from build123d import *

# Parameters (mm, degrees)
BOSS_EXTRUDE1_DEPTH = 1.5875
SKETCH2_R           = 13.081
CUT_EXTRUDE1_DEPTH  = 282.7782
CUT_EXTRUDE2_REACH  = 907.396
SKETCH3_R           = 13.081
SKETCH5_RX          = 13.458967046
SKETCH5_RY          = 13.27706685
CUT_EXTRUDE3_DEPTH  = 850.411898389
SKETCH7_RX          = 13.827169688
SKETCH7_RY          = 13.509347203
CUT_EXTRUDE4_DEPTH  = 850.411898525
SURFACECUT1_ANGLE   = 12.730551
CUT_EXTRUDE13_DEPTH = 850.411898527
CUT_EXTRUDE14_START = -3.175
CUT_EXTRUDE14_DEPTH = 3.175
CUT_EXTRUDE15_DEPTH = 850.411898527
CUT_EXTRUDE16_DEPTH = 850.411898527
FILLET1_R           = 25.4
SKETCH28_W          = 101.6
SKETCH28_H          = 1.7907
CUT_EXTRUDE17_DEPTH = 850.411898527
CUT_EXTRUDE18_DEPTH = 850.411898527
CUT_EXTRUDE19_DEPTH = 850.411898527


# Read off the part's stored shape, not the designer's step: SurfaceCut1, Cut-Extrude14
with BuildPart() as part:
    # Sketch1 → Boss-Extrude1 (new, symmetric)
    with BuildSketch(Plane(origin=(-71.4375, 0, 0), x_dir=(0, 0, -1), z_dir=(1, 0, 0))):
        Polygon((139.7, -400.05), (29.21, -400.05), (29.21, -76.2), (-154.94, -76.2), (-154.94, -389.89), (-262.89, -389.89), (-262.89, -76.2), (-384.81, -76.2), (-384.81, -342.9), (-454.66, -342.9), (-454.66, -76.2), (-749.3, -76.2), (-749.3, 76.2), (-454.66, 76.2), (-454.66, 342.9), (-384.81, 342.9), (-384.81, 76.2), (-262.89, 76.2), (-262.89, 389.89), (-154.94, 389.89), (-154.94, 76.2), (29.21, 76.2), (29.21, 400.05), (139.7, 400.05), (139.7, 92.075), (107.95, 92.075), (107.95, 88.9), (139.7, 88.9), (139.7, -88.9), (107.95, -88.9), (107.95, -92.075), (139.7, -92.075), align=None)
    extrude(amount=BOSS_EXTRUDE1_DEPTH, both=True)

    # Sketch2 → Cut-Extrude1 (cut)
    with BuildSketch(Plane(origin=(209.7532, 370.332, -29.3624), x_dir=(0, 0, -1), z_dir=(1, 0, 0))):
        Circle(SKETCH2_R)
    cut_extrude1 = extrude(amount=-CUT_EXTRUDE1_DEPTH, mode=Mode.SUBTRACT)

    # Cut-Extrude2: up to this plane
    cut_extrude2_end = Plane(origin=(-73.025, 0, 0), z_dir=(-1, 0, 0))
    # Sketch3 → Cut-Extrude2 (cut, up to the surface)
    with BuildSketch(Plane(origin=(4.654591859, 367.519252147, 275.4376), x_dir=(0.13291538281760473, 0.03562595760229639, -0.9904868965086662), z_dir=(0.9567163781525703, 0.25643335182849597, 0.13760707774177544)), mode=Mode.PRIVATE) as cut_extrude2_sk1:
        Circle(SKETCH3_R)
    cut_extrude2_tool1 = split(extrude(cut_extrude2_sk1.sketch, amount=-CUT_EXTRUDE2_REACH, mode=Mode.PRIVATE), bisect_by=cut_extrude2_end, keep=Keep.BOTH, mode=Mode.PRIVATE)
    cut_extrude2 = cut_extrude2_tool1.solids().sort_by_distance((4.654592, 367.519252, 275.4376))[0]
    add(cut_extrude2, mode=Mode.SUBTRACT)

    # Sketch5 → Cut-Extrude3 (cut, through all)
    with BuildSketch(Plane(origin=(-69.85, 0, 0), x_dir=(0, 0, -1), z_dir=(1, 0, 0))):
        with Locations(Location((-264.721405109, 347.549423415), (0, 0, 82.179315893))):
            Ellipse(SKETCH5_RX, SKETCH5_RY)
    cut_extrude3 = extrude(amount=-CUT_EXTRUDE3_DEPTH, mode=Mode.SUBTRACT)

    # Sketch7 → Cut-Extrude4 (cut, through all)
    with BuildSketch(Plane.ZY.offset(73.025)):
        with Locations(Location((264.264736359, 346.698412696), (0, 0, -95.705935517))):
            Ellipse(SKETCH7_RX, SKETCH7_RY)
    cut_extrude4 = extrude(amount=-CUT_EXTRUDE4_DEPTH, mode=Mode.SUBTRACT)

    # SurfaceCut1 outline → SurfaceCut1 (revolve, cut)
    with BuildSketch(Plane(origin=(-25.4, 215.408274925, 0), x_dir=(-0.43753517000423214, 0.899201298380606, 0), z_dir=(0.899201298380606, 0.43753517000423214, 0))):
        with BuildLine():
            ThreePointArc((76.208166822, 454.660000025), (88.899999997, 442.415379638), (101.591833177, 454.660000021))
            Line((101.591833177, 454.660000021), (76.208166822, 454.660000025))
        make_face()
    surfacecut1 = revolve(axis=Axis((-25.4, 215.408274925, 0), (0, 0, 1)), revolution_arc=SURFACECUT1_ANGLE, mode=Mode.SUBTRACT)

    # Sketch21 → Cut-Extrude13 (cut, through all)
    with BuildSketch(Plane.ZY.offset(73.025)):
        with BuildLine():
            Line((454.66, 303.637577447), (454.66, 274.279071706))
            ThreePointArc((454.66, 274.279071706), (442.249689548, 288.958324577), (454.66, 303.637577447))
        make_face()
    cut_extrude13 = extrude(amount=-CUT_EXTRUDE13_DEPTH, mode=Mode.SUBTRACT)

    # Cut-Extrude14 outline → Cut-Extrude14 (cut)
    with BuildSketch(Plane(origin=(-69.85, 0, 0), x_dir=(0, 0, -1), z_dir=(1, 0, 0)).offset(CUT_EXTRUDE14_START)):
        with BuildLine():
            Line((-454.66, 291.370782877), (-442.446465515, 291.370782877))
            add(Edge.make_bspline(
                [(-442.446465515, 291.370782877), (-442.305604528, 293.829318521), (-442.944960374, 298.079765742), (-445.927339463, 302.763682225), (-449.764908378, 305.786294337), (-452.799544613, 306.691151874), (-454.66, 306.759783223)],
                knots=[0, 0, 0, 0, 0.33604966, 0.578754716, 0.743869723, 1, 1, 1, 1], degree=3))
            Line((-454.66, 306.759783223), (-454.66, 291.370782877))
        make_face()
    cut_extrude14 = extrude(amount=CUT_EXTRUDE14_DEPTH, mode=Mode.SUBTRACT)

    # Sketch25 → Cut-Extrude15 (cut, through all)
    with BuildSketch(Plane(origin=(-69.85, 0, 0), x_dir=(0, 0, -1), z_dir=(1, 0, 0))):
        with BuildLine():
            Line((-442.434347234, 291.295796674), (-456.435114382, 293.070911057))
            Line((-456.435114382, 293.070911057), (-454.66, 307.071678205))
            ThreePointArc((-454.66, 307.071678205), (-445.279881573, 301.715753032), (-442.434347234, 291.295796674))
        make_face()
    cut_extrude15 = extrude(amount=-CUT_EXTRUDE15_DEPTH, mode=Mode.SUBTRACT)

    # Sketch27 → Cut-Extrude16 (cut, through all)
    with BuildSketch(Plane(origin=(-69.85, 0, 0), x_dir=(0, 0, -1), z_dir=(1, 0, 0))):
        with BuildLine():
            Line((-443.216925762, 283.679849678), (-443.400538268, 298.481302661))
            ThreePointArc((-443.400538268, 298.481302661), (-441.972420297, 291.09715316), (-443.216925762, 283.679849678))
        make_face()
    cut_extrude16 = extrude(amount=-CUT_EXTRUDE16_DEPTH, mode=Mode.SUBTRACT)

    # Mirror1: Cut-Extrude1, Cut-Extrude2, Cut-Extrude3, Cut-Extrude4, SurfaceCut1, Cut-Extrude13, Cut-Extrude14, Cut-Extrude15, Cut-Extrude16 across plane
    add(cut_extrude1.mirror(Plane.ZX), mode=Mode.SUBTRACT)
    add(cut_extrude2.mirror(Plane.ZX), mode=Mode.SUBTRACT)
    add(cut_extrude3.mirror(Plane.ZX), mode=Mode.SUBTRACT)
    add(cut_extrude4.mirror(Plane.ZX), mode=Mode.SUBTRACT)
    add(surfacecut1.mirror(Plane.ZX), mode=Mode.SUBTRACT)
    add(cut_extrude13.mirror(Plane.ZX), mode=Mode.SUBTRACT)
    add(cut_extrude14.mirror(Plane.ZX), mode=Mode.SUBTRACT)
    add(cut_extrude15.mirror(Plane.ZX), mode=Mode.SUBTRACT)
    add(cut_extrude16.mirror(Plane.ZX), mode=Mode.SUBTRACT)

    # Fillet1
    fillet1_edges = [part.edges().sort_by_distance(p)[0] for p in [
        (-71.4375, -76.2, -29.21),
        (-71.4375, -76.2, 154.94),
        (-71.4375, -76.2, 262.89),
        (-71.4375, -76.2, 454.66),
        (-71.4375, 76.2, 454.66),
        (-71.4375, 76.2, 262.89),
        (-71.4375, 76.2, 154.94),
        (-71.4375, 76.2, -29.21),
    ]]
    fillet(fillet1_edges, radius=FILLET1_R)

    # Sketch28 → Cut-Extrude17 (cut, through all)
    with BuildSketch(Plane(origin=(-69.85, 0, 0), x_dir=(0, 0, -1), z_dir=(1, 0, 0))):
        with Locations((-698.5, -0.89535)):
            Rectangle(SKETCH28_W, SKETCH28_H)
        with Locations((-698.5, 0.89535)):
            Rectangle(SKETCH28_W, SKETCH28_H)
    extrude(amount=-CUT_EXTRUDE17_DEPTH, mode=Mode.SUBTRACT)

    # Sketch29 → Cut-Extrude18 (cut, through all)
    with BuildSketch(Plane(origin=(-69.85, 0, 0), x_dir=(0, 0, -1), z_dir=(1, 0, 0))):
        Polygon((29.21, 118.85525736), (41.91, 118.85525736), (41.91, 96.357238024), (28.663036975, 96.357238024), align=None)
        Polygon((29.21, -118.85525736), (41.91, -118.85525736), (41.91, -96.357238024), (28.663036975, -96.357238024), align=None)
    extrude(amount=-CUT_EXTRUDE18_DEPTH, mode=Mode.SUBTRACT)

    # Sketch30 → Cut-Extrude19 (cut, through all)
    with BuildSketch(Plane(origin=(-69.85, 0, 0), x_dir=(0, 0, -1), z_dir=(1, 0, 0))):
        with BuildLine():
            Line((-231.14, 389.89), (-231.14, 364.49))
            ThreePointArc((-231.14, 364.49), (-205.74, 339.09), (-180.34, 364.49))
            Line((-180.34, 364.49), (-180.34, 389.89))
            Line((-180.34, 389.89), (-231.14, 389.89))
        make_face()
    cut_extrude19 = extrude(amount=-CUT_EXTRUDE19_DEPTH, mode=Mode.SUBTRACT)

    # Mirror2: Cut-Extrude19 across plane
    add(cut_extrude19.mirror(Plane.ZX), mode=Mode.SUBTRACT)


solid = part.part
Can you work these out from the model? Positions are in its coordinate system, mm. A direction names the side the tool comes from. Coordinates: 2 decimals unless noted, no trailing zeros. Write each loop counter-clockwise with the first axis right and the second up, starting at its lowest first coordinate (ties: lowest second). Pieces come first, ordered by that corner, then holes. Notation, with made-up numbers: (88.5, -28.75) -> (123.5, -28.75) arc R11 ccw to (123.5, -20.75) -> close; hole circle Ø7 at (44.25, -12). An arc over 180 degrees is marked (long way). Write each question's results on one line, items separated by ' | '. Start each with the question number.
Q1. Imagine slicing it at A-A (y = -204). Write out the boundary of the cut face in (x, z) (3 decimals), then the cut area to 3 significant figures.
Q2. I'm going to push flat-ended pins straight in: pin 1 (1 mm diameter, centred on x = -71, y = 195, fed in from +Z); pin 2 (1.5 mm diameter, centred on x = -70.5, z = 92.5, fed in from -Y); pin 3 (1 mm diameter, centred on x = -71, z = 713.5, fed in from +Y). Where does each tip first touch, or does it pass through?
Q3. Imagine slicing it at B-B (z = 219.5). Write out the boundary of the cut face in (x, y) (3 decimals), then the cut area to 3 significant figures.
Q4. We'd pull the mould along Z, two halves only. Please class faces 4 (the face through (-71.46, -83.44, 270.53)), 5 (the face through (-71.46, 83.84, 461.9)), 6 (the face through (-73.025, 2, 237)): +Z half, -Z half, draft (parallel to the pull), parting line (faces both ways), or undercut.
Q5. If I drill on probe 1 along Z at (x, y) = (-72.35, -311.5); probe 2 along Z at (x, y) = (-71.55, -291); probe 3 along Y at (x, z) = (-72.6, 712), over which ranges is the centre line in solid material (lowest first)?
Q6. On a 3-axis mill with a long thin cutter (end or side, diameter ignored), from which of +Z, -Z, +X, -X, +Y, -Y can I reach the whole of each face in a straight line? I mean faces 1 (the face through (-71.46, -83.84, 147.7)), 2 (the face through (-71.46, 83.44, 147.3)), 3 (the face through (-71.46, -83.44, 462.3)). Say none if no direction works.
Taken from the geometry:
1) outline: (-73.025, -139.7) -> (-69.85, -139.7) -> (-69.85, -29.21) -> (-73.025, -29.21) -> close; (-73.025, 154.94) -> (-69.85, 154.94) -> (-69.85, 262.89) -> (-73.025, 262.89) -> close; (-73.025, 384.81) -> (-69.85, 384.81) -> (-69.85, 454.66) -> (-73.025, 454.66) -> close | area: 915 mm^2
2) pin 1: stops at z = 454.66 | pin 2: stops at y = -76.2 | pin 3: stops at y = 76.2
3) outline: (-73.025, -343.14) -> (-69.85, -343.14) -> (-69.85, 343.14) -> (-73.025, 343.14) -> close | area: 2,180 mm^2
4) face 4: undercut | face 5: +Z half | face 6: draft
5) probe 1: z = -139.7 to -29.21, 154.94 to 262.89, 384.81 to 454.66 | probe 2: z = -139.7 to -29.21, 154.94 to 262.89, 384.81 to 441.97 | probe 3: y = -76.2 to -1.79, 1.79 to 76.2
6) face 1: +X, -X, -Y | face 2: +X, -X, +Y | face 3: +Z, +X, -X, -Y
